Autodesk Inventor part; units mm, degrees
ref_plane "YZ Plane" through (0, 0, 0) normal (1, 0, 0) x (0, 1, 0)
ref_plane "XZ Plane" through (0, 0, 0) normal (0, 1, 0) x (-1, 0, 0)
ref_plane "XY Plane" through (0, 0, 0) normal (0, 0, 1) x (1, 0, 0)
sketch "スケッチ1" plane through (0, 0, 0) normal (0, 1, 0) x (-1, 0, 0)
  line L0 (7.5, 7.5) -> (-7.5, 7.5)
  line L1 (-7.5, 7.5) -> (-7.5, -7.5)
  line L2 (-7.5, -7.5) -> (7.5, -7.5)
  line L3 (7.5, -7.5) -> (7.5, 7.5)
  line L4 (7.5, 7.5) -> (-7.5, -7.5) construction
  line L5 (-7.5, 7.5) -> (7.5, -7.5) construction
  line L6 (5, 3) -> (-5, 3)
  line L7 (-5, 3) -> (-5, -3)
  line L8 (-5, -3) -> (5, -3)
  line L9 (5, -3) -> (5, 3)
  line L10 (5, 3) -> (-5, -3) construction
  line L11 (-5, 3) -> (5, -3) construction
  point P0 (0, 0)
  dimension "d0" = 15
  dimension "d1" = 15
  dimension "d2" = 10
  dimension "d3" = 6
extrude "押し出し1" add sketch "スケッチ1" along normal blind 2
sketch "スケッチ2" plane through (0, 2, 0) normal (0, 1, 0) x (1, 0, 0)
  line L0 (-6.75, 2.15) -> (6.75, 2.15)
  line L1 (6.75, 2.15) -> (6.75, -2.15)
  line L2 (6.75, -2.15) -> (-6.75, -2.15)
  line L3 (-6.75, -2.15) -> (-6.75, 2.15)
  line L4 (-6.75, 2.15) -> (6.75, -2.15) construction
  line L5 (6.75, 2.15) -> (-6.75, -2.15) construction
  line L6 (-5, -3) -> (-5, 3)
  line L7 (-5, 2.15) -> (-5, -2.15)
  line L8 (5, 3) -> (5, -3)
  line L9 (5, 2.15) -> (5, -2.15)
  point P0 (0, 0)
  dimension "d8" = 13.5
  dimension "d9" = 4.3
extrude "押し出し2" add sketch "スケッチ2" along normal blind 7 contours L0 L6 L2 L3 | L0 L1 L2 L8
fillet "フィレット1" radius 2 2 edges at (6.75, 2, 0) (-6.75, 2, 0)
fillet "フィレット2" radius 2 4 edges at (-7.5, 1, 7.5) (7.5, 1, 7.5) (7.5, 1, -7.5) (-7.5, 1, -7.5)
properties part number "LRA_case3"
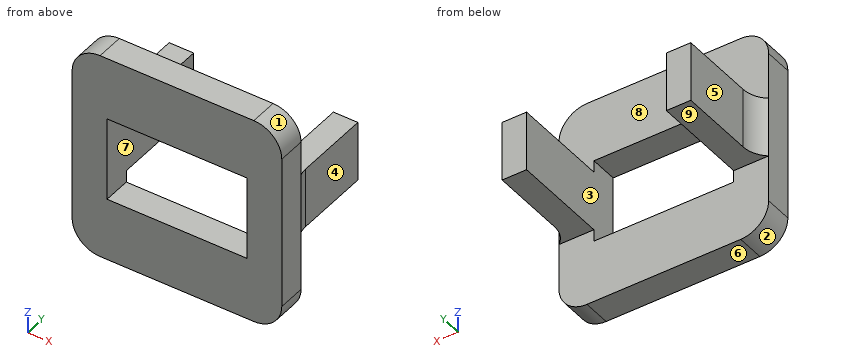
Can you work these out from the model? Positions are in its coordinate system, mm. Face numbers are marked on the shaded views. A direction names the side the tool comes from. Give positions to 0.01 mm unless a question says otherwise; leave off trailing zeros. Loops run counter-clockwise (first coordinate to the right, second up) from the corner with the lowest first, then second, coordinate; pieces in that order, holes last. Notation, with made-up numbers: M -35,70 L 18,70 A18 ccw 18,86 Z; hole C 0,33 d10. An arc over 180 degrees is marked long. One line per item, written item: value. Start each with the question number.
1) Thinking about a two-plate mould opening in Z: for the marked faces 1, 2, 3 and 4, which applies, +Z half, -Z half, draft (parallel to the pull), parting line (faces both ways), or undercut?
2) If we section it at B-B, the plane x = 2: Write out the boundary of the cut face in (y, z), and give its area (3 significant figures).
3) On a 3-axis mill with a long thin cutter (end or side, diameter ignored), from which of +Z, -Z, +X, -X, +Y, -Y can I reach the whole of each face in a straight line? I mean the marked faces 5, 6, 7, 8 and 9. Say none if no direction works.
4) I'm going to push flat-ended pins straight in: pin 1 (2 mm diameter, centred on x = -6.5, y = 6.5, fed in from -Z); pin 2 (8 mm diameter, centred on x = -4.5, z = 0.5, fed in from +Y); pin 3 (6 mm diameter, centred on x = -1.5, z = -5, fed in from +Y); pin 4 (2 mm diameter, centred on y = 5.5, z = -1, fed in from +X). Where does each tip first touch, or does it pass through?
5) If I drill on line 1 (X direction, y = 3.75, z = 1.5); line 2 (Z direction, x = -3, y = 1.5); line 3 (Y direction, x = -0.25, z = -5), over which ranges is the centre line in solid material (lowest first)? Write a range as [from, to].
6) If we section it at C-C, the plane y = 1.25: Write out the boundary of the cut face in (x, z), and give its area (3 significant figures).
7) If we section it at D-D, the plane x = -5.75: Write out the boundary of the cut face in (y, z), and give its area (3 significant figures).
8) If we section it at A-A, the plane y = 6.75: Write out the boundary of the cut face in (x, z).
Completed:
1. face 1: +Z half
1. face 2: -Z half
1. face 3: undercut
1. face 4: draft
2. outline: M 0,-7.5 L 2,-7.5 L 2,-3 L 0,-3 Z; M 0,3 L 2,3 L 2,7.5 L 0,7.5 Z
2. area: 18.0 mm^2
3. face 5: +Z, -Z, -X, +Y
3. face 6: -Z, +X, -X, +Y, -Y
3. face 7: +Y, -Y
3. face 8: +Z, +X, -X, +Y
3. face 9: -Z, +X, -X, +Y
4. pin 1: stops at z = -2.15
4. pin 2: stops at y = 9
4. pin 3: stops at y = 2
4. pin 4: stops at x = 6.75
5. line 1: x = [-6.75, -5], [5, 6.75]
5. line 2: z = [-7.5, -3], [3, 7.5]
5. line 3: y = [0, 2]
6. outline: M -7.5,-5.5 A2 ccw -5.5,-7.5 L 5.5,-7.5 A2 ccw 7.5,-5.5 L 7.5,5.5 A2 ccw 5.5,7.5 L -5.5,7.5 A2 ccw -7.5,5.5 Z; hole M -5,-3 L 5,-3 L 5,3 L -5,3 Z
6. area: 162 mm^2
7. outline: M 0,-7.48 L 2,-7.48 L 2,-2.15 L 9,-2.15 L 9,2.15 L 2,2.15 L 2,7.48 L 0,7.48 Z
7. area: 60.0 mm^2
8. outline: M -6.75,-2.15 L -5,-2.15 L -5,2.15 L -6.75,2.15 Z; M 5,-2.15 L 6.75,-2.15 L 6.75,2.15 L 5,2.15 Z
